Autodesk Inventor part; units mm, degrees
ref_plane "YZ Plane" through (0, 0, 0) normal (1, 0, 0) x (0, 1, 0)
ref_plane "XZ Plane" through (0, 0, 0) normal (0, 1, 0) x (-1, 0, 0)
ref_plane "XY Plane" through (0, 0, 0) normal (0, 0, 1) x (1, 0, 0)
sketch "Sketch1" plane through (0, 0, 0) normal (0, 0, 1) x (1, 0, 0)
  line L0 (-1.7679, 0.1299) -> (-1.7679, -25.6595)
  line L1 (-1.7679, -25.6595) -> (3, -25.6595)
  line L2 (3, -25.6595) -> (3, -15.6595)
  line L3 (3, -15.6595) -> (0, -15.6595)
  line L4 (0, -15.6595) -> (0, 0.1299)
  line L5 (-1.7679, 0.1299) -> (0, 0.1299)
  circle A0 centre (0, -18.6595) radius 1.5
  line L6 (-5.2321, -25.6595) -> (-5.2321, 0.1299)
  line L7 (-10, 0.1299) -> (-5.2321, 0.1299)
  line L8 (-10, -25.6595) -> (-10, 0.1299)
  line L9 (-10, -25.6595) -> (-5.2321, -25.6595)
  circle A1 centre (-7, -22.6595) radius 1.5
  line L10 (3, -25.6595) -> (-10, -25.6595)
  line L11 (-10, -25.6595) -> (-10, -15.6595)
  line L12 (-10, -15.6595) -> (3, -15.6595)
  line L13 (3, -15.6595) -> (3, -25.6595)
  point P0 (0, 0)
extrude "Extrusion1" add sketch "Sketch1" along normal blind 6 contours L12 L3 L2 L1 L0 | L0 L10 L6 L12 | L6 L9 L8 L12
sketch "Sketch2" plane through (-10, -25.6595, 0) normal (0, -1, 0) x (1, 0, 0)
  line L0 (0, 0) -> (13, 0)
  line L1 (13, 0) -> (13, 6)
  line L2 (0, 6) -> (13, 6)
  line L3 (0, 0) -> (0, 6)
  arc A0 (4.7679, 0) -> (8.2321, 0) centre (6.5, 1) ccw
  line L4 (0, 0) -> (4.7679, 0)
  line L5 (0, 0) -> (0, -4)
  line L6 (0, -4) -> (13, -4)
  line L7 (13, 0) -> (13, -4)
  line L8 (8.2321, 0) -> (13, 0)
  circle A1 centre (6.5, 0.5) radius 2
  point P0 (10, 0)
  dimension "d2" = 4
  dimension "d3" = 6.5
  dimension "d4" = 0.5
extrude "Extrusion2" cut sketch "Sketch2" against normal through all contours L0 A1 | A0 L0 A1
properties part number "eye_cam_clamp"
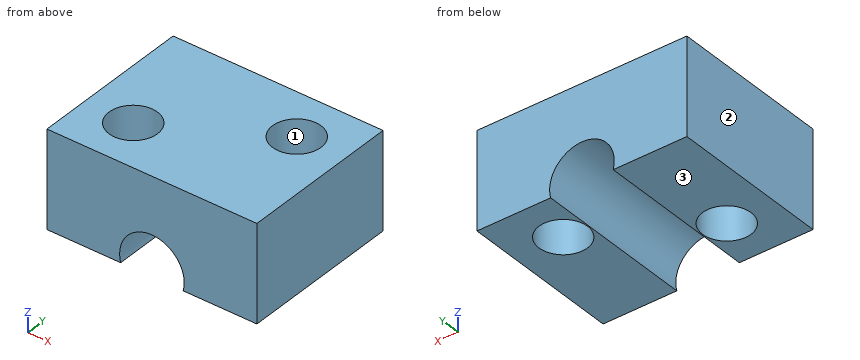
Geometry check sheet. Reference: the model listing, model coordinates, mm. Face numbers are marked on the shaded views. Coordinates: 2 decimals unless noted, no trailing zeros. Loops run counter-clockwise (first coordinate to the right, second up) from the corner with the lowest first, then second, coordinate; pieces in that order, holes last. Notation, with made-up numbers: (45, 6.5) - (73, 6.5) arc R20 ccw to (73, 11.5) - close; hole circle Ø11 at (31, 61.25). An arc over 180 degrees is marked (long way). One line per item, written item: value. Start each with the question number.
(1) Cross-section at A-A on z = 2. Enter the section's corners in (x, y), plus the area to 3 significant figures.
(2) Material ranges on line 1 (X direction, y = -20, z = 1.25); line 2 (Y direction, x = 0, z = 1.8); line 3 (X direction, y = -24, z = 1.65), recorded low to high. Write a range as [from, to].
(3) Cross-section at D-D on z = 1.3. Enter the section's corners in (x, y), plus the area to 3 significant figures.
(4) Cross-section at C-C on y = -17.5. Enter the section's corners in (x, z), plus the area to 3 significant figures.
(5) Cross-section at B-B on x = 0. Enter the section's corners in (y, z), plus the area to 3 significant figures.
(6) Depth check by flat-ended pin: P1, Ø3.5, axis at x = -7, y = -22.66, coming from the +Z side; P2, Ø2, axis at x = -4, y = -17.5, coming from the -Z side. Enter the tip coordinate at first touch or a pass-through.
(7) Mould release check, pull along X, two halves, no side actions. Record for the marked faces 1, 2 and 3: released by +X, released by -X, zero draft, split by the parting line, or undercut.
Results below:
1. outline: (-10, -25.66) - (-4.82, -25.66) - (-4.82, -15.66) - (-10, -15.66) - close; (-2.18, -25.66) - (3, -25.66) - (3, -15.66) - (-2.18, -15.66) - close; hole circle Ø3 at (-7, -22.66); hole circle Ø3 at (0, -18.66)
1. area: 89.4 mm2
2. line 1: x = [-10, -5.35], [-1.65, -0.67], [0.67, 3]
2. line 2: y = [-25.66, -20.16], [-17.16, -15.66]
2. line 3: x = [-10, -7.67], [-6.33, -5.14], [-1.86, 3]
3. outline: (-10, -25.66) - (-5.33, -25.66) - (-5.33, -15.66) - (-10, -15.66) - close; (-1.67, -25.66) - (3, -25.66) - (3, -15.66) - (-1.67, -15.66) - close; hole circle Ø3 at (-7, -22.66); hole circle Ø3 at (0, -18.66)
3. area: 79.2 mm2
4. outline: (-10, 0) - (-5.44, 0) arc R2 cw (long way) to (-1.56, 0) - (-0.95, 0) - (-0.95, 6) - (-10, 6) - close; (0.95, 0) - (3, 0) - (3, 6) - (0.95, 6) - close
4. area: 58.3 mm2
5. outline: (-25.66, 0) - (-20.16, 0) - (-20.16, 6) - (-25.66, 6) - close; (-17.16, 0) - (-15.66, 0) - (-15.66, 6) - (-17.16, 6) - close
5. area: 42.0 mm2
6. P1: stops at z = 6
6. P2: stops at z = 1.82
7. face 1: undercut
7. face 2: released by -X
7. face 3: zero draft
